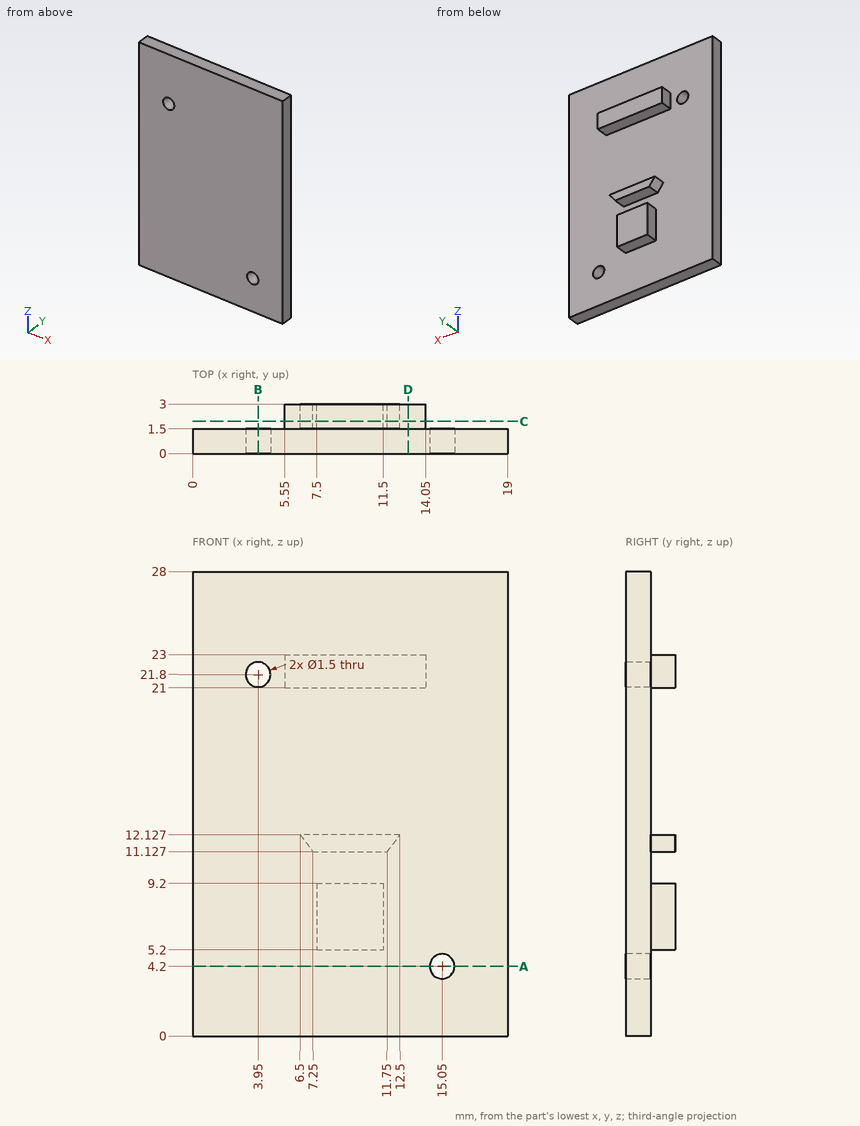
Job drawing, mm, ordinate dimensions from the low corner. One solid piece. Give positions to 0.01 mm unless a question says otherwise; leave off trailing zeros. Write each loop counter-clockwise with the first axis right and the second up, starting at its lowest first coordinate (ties: lowest second). Pieces come first, ordered by that corner, then holes. Notation, with made-up numbers: M 17.25,88.25 L 76.25,88.25 A7 ccw 76.25,93.25 Z; hole C 4,-22.5 d7. An arc over 180 degrees is marked long. One line per item, written item: value. Start each with the question number.
Q1. Saw through at C-C, the plane y = 1.95. Write the cut outline in (x, z).
Q2. Saw through at A-A, the plane z = 4.2. Write the cut outline in (x, y).
Q3. Drop flat-ended pins along their axis: pin 1 Ø0.9 at (x, z) = (15.05, 4.2) entering from +Y; pin 2 Ø1.2 at (x, y) = (9.5, 2.5) entering from +Z; pin 3 Ø1.7 at (x, z) = (3.95, 21.8) entering from +Y; pin 4 Ø0.8 at (y, z) = (2.5, 22.5) entering from +X. Give the stop position or say it passes through.
Q4. Saw through at D-D, the plane x = 13. Write the cut outline in (y, z), plus the area to 3 significant figures.
Q5. Saw through at B-B, the plane x = 3.95. Write the cut outline in (y, z).
Q6. Probe probe 1 along X at (y, z) = (1.15, 21.8); probe 2 along X at (y, z) = (1, 4.2); probe 3 along Y at (x, z) = (14.25, 12). List the from-to ranges inside material, lowest first. Write a range as [from, to].
Output values:
1. outline: M 5.55,21 L 14.05,21 L 14.05,23 L 5.55,23 Z; M 6.5,12.13 L 7.25,11.13 L 11.75,11.13 L 12.5,12.13 Z; M 7.5,5.2 L 11.5,5.2 L 11.5,9.2 L 7.5,9.2 Z
2. outline: M 0,0 L 14.3,0 L 14.3,1.5 L 0,1.5 Z; M 15.8,0 L 19,0 L 19,1.5 L 15.8,1.5 Z
3. pin 1: passes through
3. pin 2: stops at z = 23
3. pin 3: stops at y = 1.5
3. pin 4: stops at x = 14.05
4. outline: M 0,0 L 1.5,0 L 1.5,21 L 3,21 L 3,23 L 1.5,23 L 1.5,28 L 0,28 Z
4. area: 45.0 mm²
5. outline: M 0,0 L 1.5,0 L 1.5,21.05 L 0,21.05 Z; M 0,22.55 L 1.5,22.55 L 1.5,28 L 0,28 Z
6. probe 1: x = [0, 3.2], [4.7, 19]
6. probe 2: x = [0, 14.3], [15.8, 19]
6. probe 3: y = [0, 1.5]
